The listing builds one solid part. Answer for the finished solid, in the listing's coordinates (mm). Round coordinates to 2 decimals unless told otherwise and drop trailing zeros. Write each loop counter-clockwise with the first axis right and the second up, starting at its lowest first coordinate (ties: lowest second). Pieces come first, ordered by that corner, then holes.
Item 1: Find section A-A on y = -102. Give the vertices of the cut face in (x, z).
Item 2: Find section B-B on z = 1.95. Give the vertices of the cut face in (x, y), then the cut area to 3 significant figures.
Item 3: Find the intervals of material crossed by probe 1 along X at (y, z) = (-69.5, 3.9); probe 2 along Y at (x, z) = (-56, 3.6); probe 3 along Y at (x, z) = (-55, 2), in increasing order.
Item 4: Each of these flat-tipped pins is pushed along its axis until it touches: pin 1 (2 mm diameter, centred on y = 77.5, z = 2.5, fed in from -X); pin 2 (5 mm diameter, centred on x = 30.95, y = -102, fed in from +Z); pin 3 (1.5 mm diameter, centred on x = -160, z = 3, fed in from +Y). Where does it stop, or does it pass through?
Item 5: Find section C-C on y = -0.5. Give the vertices of the cut face in (x, z), then the cut area to 3 significant figures.
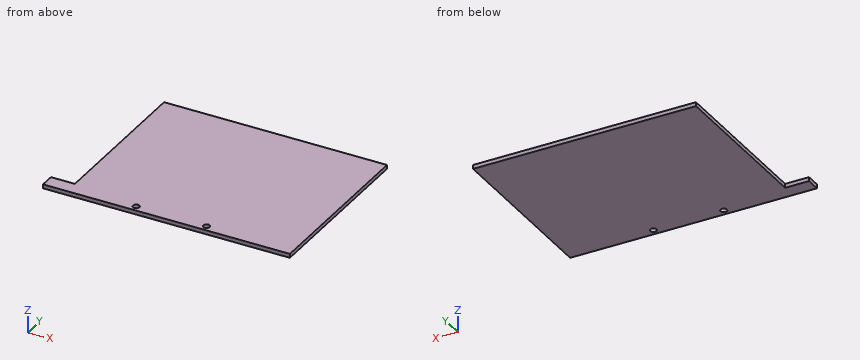
```python
from build123d import *

# Parameters (mm, degrees)
SKETCH1_W           = 280
SKETCH1_H           = 220
SKETCH1_W_2         = 30
SKETCH1_H_2         = 18
BOSS_EXTRUDE1_DEPTH = 5
SKETCH2_R           = 4
CUT_EXTRUDE1_DEPTH  = 10


with BuildPart() as part:
    # Sketch1 → Boss-Extrude1 (new body)
    with BuildSketch(Plane.XY):
        Rectangle(SKETCH1_W, SKETCH1_H)
        with Locations((-155, -101)):
            Rectangle(SKETCH1_W_2, SKETCH1_H_2)
    extrude(amount=BOSS_EXTRUDE1_DEPTH)

    # Sketch2 → Cut-Extrude1 (cut)
    with BuildSketch(Plane.XY.offset(5)):
        with Locations((-57.377117084, -102)):
            Circle(SKETCH2_R)
        with Locations((30.950491695, -102)):
            Circle(SKETCH2_R)
    extrude(amount=-CUT_EXTRUDE1_DEPTH, mode=Mode.SUBTRACT)


solid = part.part
```
Check values:
1. outline: (-170, 0) - (-61.38, 0) - (-61.38, 5) - (-170, 5) - close; (-53.38, 0) - (26.95, 0) - (26.95, 5) - (-53.38, 5) - close; (34.95, 0) - (140, 0) - (140, 5) - (34.95, 5) - close
2. outline: (-170, -110) - (140, -110) - (140, 110) - (-140, 110) - (-140, -92) - (-170, -92) - close; hole circle Ø8 at (-57.38, -102); hole circle Ø8 at (30.95, -102)
2. area: 62,000 mm2
3. probe 1: x = -140 to 140
3. probe 2: y = -110 to -105.76, -98.24 to 110
3. probe 3: y = -110 to -105.22, -98.78 to 110
4. pin 1: stops at x = -140
4. pin 2: passes through
4. pin 3: stops at y = -92
5. outline: (-140, 0) - (140, 0) - (140, 5) - (-140, 5) - close
5. area: 1,400 mm2
